```python
from build123d import *

# Parameters (mm, degrees)
BOSS_EXTRUDE1_DEPTH = 8.255
FILLET1_R           = 4.191
SKETCH2_R           = 2.07899
CUT_EXTRUDE1_DEPTH  = 81.896006892
FILLET2_R           = 4.191
SKETCH3_R           = 2.07899
CUT_EXTRUDE2_DEPTH  = 8.255


with BuildPart() as part:
    # Sketch1 → Boss-Extrude1 (new body)
    with BuildSketch(Plane(origin=(0, 0, 0), x_dir=(1, 0, 0), z_dir=(0, 1, 0))):
        Polygon((69.85, -8.001), (69.85, -9.99998), (0, -9.99998), (0, -8.001), (9.99998, -8.001), (9.99998, -1.99898), (0, -1.99898), (0, 0), (69.85, 0), (69.85, -1.99898), (79.84998, -1.99898), (79.84998, -8.001), align=None)
    extrude(amount=BOSS_EXTRUDE1_DEPTH)

    # Fillet1
    # the kernel refuses this fillet: 4.191 mm, written as the material it takes off along each edge
    with BuildSketch(Plane(origin=(0, 0, 12.47648), x_dir=(0, 1, 0), z_dir=(0, 0, -1)), Plane(origin=(0, 0, 20.47748), x_dir=(0, 1, 0), z_dir=(0, 0, -1))) as fillet1_piece_1:
        with BuildLine():
            CenterArc((FILLET1_R, FILLET1_R), FILLET1_R, 180, 90)
            Line((0, FILLET1_R), (0, 0))
            Line((0, 0), (FILLET1_R, 0))
        make_face()
    extrude(amount=22.95398, mode=Mode.SUBTRACT)
    with BuildSketch(Plane(origin=(0, 8.255, 12.47648), x_dir=(0, -1, 0), z_dir=(0, 0, -1)), Plane(origin=(0, 8.255, 20.47748), x_dir=(0, -1, 0), z_dir=(0, 0, -1))) as fillet1_piece_2:
        with BuildLine():
            CenterArc((FILLET1_R, -FILLET1_R), FILLET1_R, 90, 90)
            Line((0, -FILLET1_R), (0, 0))
            Line((0, 0), (FILLET1_R, 0))
        make_face()
    extrude(amount=22.95398, mode=Mode.SUBTRACT)

    # Sketch2 → Cut-Extrude1 (cut, through all)
    with BuildSketch(Plane.XY.offset(9.99998)):
        with Locations((2.587471088, 4.1275)):
            Circle(SKETCH2_R)
    extrude(amount=-CUT_EXTRUDE1_DEPTH, mode=Mode.SUBTRACT)

    # Fillet2
    # the kernel refuses this fillet: 4.191 mm, written as the material it takes off along each edge
    with BuildSketch(Plane(origin=(79.84998, 0, -8.47852), x_dir=(-1, 0, 0), z_dir=(0, 0, 1))) as fillet2_piece_1:
        with BuildLine():
            CenterArc((FILLET2_R, -FILLET2_R), FILLET2_R, 90, 90)
            Line((0, -FILLET2_R), (0, 0))
            Line((0, 0), (FILLET2_R, 0))
        make_face()
    extrude(amount=26.95702, mode=Mode.SUBTRACT)
    with BuildSketch(Plane(origin=(79.84998, 8.255, -8.47852), x_dir=(-1, 0, 0), z_dir=(0, 0, 1))) as fillet2_piece_2:
        with BuildLine():
            CenterArc((FILLET2_R, FILLET2_R), FILLET2_R, 180, 90)
            Line((0, FILLET2_R), (0, 0))
            Line((0, 0), (FILLET2_R, 0))
        make_face()
    extrude(amount=26.95702, mode=Mode.SUBTRACT)

    # Sketch3 → Cut-Extrude2 (cut)
    with BuildSketch(Plane.XY.offset(8.001)):
        with Locations((75.65898, 4.191)):
            Circle(SKETCH3_R)
    extrude(amount=-CUT_EXTRUDE2_DEPTH, mode=Mode.SUBTRACT)


solid = part.part
```
The model under review builds one solid part; all positions refer to its coordinate system, in mm. A direction names the side the tool comes from. Give positions to 0.01 mm unless a question says otherwise; leave off trailing zeros. Write each loop counter-clockwise with the first axis right and the second up, starting at its lowest first coordinate (ties: lowest second). Pieces come first, ordered by that corner, then holes. Notation, with made-up numbers: M -6,-31 L 32,-31 A18 cw 32,-10 Z; hole C 21,87 d2. An arc over 180 degrees is marked long. Write each question's results on one line, items separated by ' | '. Start each with the question number.
1. We need section A-A (x = 74.5). Write out the cut boundary in (y, z) (3 decimals), and give its area (3 significant figures).
2. Insertion check: pin 1 Ø3.5 at (x, y) = (75.66, 4.19) entering from +Z; pin 2 Ø0.6 at (y, z) = (6, 9) entering from +X. Each pin has a flat end and moves straight along its axis. Give the tip position at first contact, or say it passes through.
3. For probe 1 along X at (y, z) = (4, 9.5); probe 2 along Z at (x, y) = (4, 6.5); probe 3 along Z at (x, y) = (73, 3.5), list the stretches that pass through material, from the lowest coordinate up. Write a range as [from, to].
4. We need section C-C (z = 5.75). Write out the cut boundary in (x, y) (1 decimal), and give its area (3 significant figures).
5. We need section B-B (y = 5). Write out the cut boundary in (x, z), and give its area (3 significant figures).
6. We need section D-D (y = 1). Write out the cut boundary in (x, z), and give its area (3 significant figures).
7. For faces 5 (the cylindrical face through (1.2, 7, 9)), 6 (the flat face through (69.85, 4, 9)), 7 (the flat face through (69.85, 4, 1)), 8 (the flat face through (10, 4, 5)), list the 3-axis set-ups (+Z, -Z, +X, -X, +Y, -Y) from which the entire face can be reached by the end or side of a thin tool; tool diameter is ignored.
8. Mouldability with a two-part tool opening along Y and no side actions: class faces 1 (the cylindrical face through (77.579, 3.395, 5.042)), 2 (the cylindrical face through (4.57, 4.75, 9.01)), 3 (the flat face through (35, 4, 10)), 4 (the cylindrical face through (78.63, 7.02, 4.96)) as released by +Y, released by -Y, zero draft, split by the parting line, or undercut.
Results found:
1) outline: M 0,1.999 L 2.465,1.999 L 2.465,8.001 L 0,8.001 Z; M 5.917,1.999 L 8.255,1.999 L 8.255,8.001 L 5.917,8.001 Z | area: 28.8 mm^2
2) pin 1: passes through | pin 2: stops at x = 69.85
3) probe 1: x = [0, 0.51], [4.66, 69.85] | probe 2: z = [0, 2], [8, 10] | probe 3: z = [2, 8]
4) outline: M 10,0 L 75.7,0 A4.2 ccw 79.8,4.1 A4.2 ccw 75.7,8.3 L 10,8.3 Z; hole C 75.7,4.2 d4.2 | area: 555 mm^2
5) outline: M 0.11,0 L 0.7,0 L 0.7,2 L 0.11,2 Z; M 0.11,8 L 0.7,8 L 0.7,10 L 0.11,10 Z; M 4.47,0 L 69.85,0 L 69.85,2 L 73.74,2 L 73.74,8 L 69.85,8 L 69.85,10 L 4.47,10 L 4.47,8 L 10,8 L 10,2 L 4.47,2 Z; M 77.57,2 L 79.74,2 L 79.74,8 L 77.57,8 Z | area: 659 mm^2
6) outline: M 1.47,0 L 69.85,0 L 69.85,2 L 78.38,2 L 78.38,8 L 69.85,8 L 69.85,10 L 1.47,10 L 1.47,8 L 10,8 L 10,2 L 1.47,2 Z | area: 684 mm^2
7) face 5: +Z, -Z, -X, +Y | face 6: +Z, +X, +Y, -Y | face 7: -Z, +X, +Y, -Y | face 8: -X, +Y, -Y
8) face 1: undercut | face 2: undercut | face 3: zero draft | face 4: released by +Y
